Design review of the part built by this model. Coordinates are the model's own, in mm. Give positions to 0.01 mm unless a question says otherwise; leave off trailing zeros. Order: outer loops, then holes, each group sorted by start corner. A loop starts at its lowest first (then second) coordinate and runs counter-clockwise, first axis right, second up.
```python
from build123d import *

# Parameters (mm, degrees)
SKETCH1_W           = 125
SKETCH1_H           = 200
BOSS_EXTRUDE1_DEPTH = 3.175
SKETCH2_R           = 2.5
CUT_EXTRUDE1_DEPTH  = 3.175
SKETCH3_R           = 6.35
CUT_EXTRUDE2_DEPTH  = 3.175


with BuildPart() as part:
    # Sketch1 → Boss-Extrude1 (new body)
    with BuildSketch(Plane.XY):
        with Locations((-62.5, 100)):
            Rectangle(SKETCH1_W, SKETCH1_H)
    extrude(amount=BOSS_EXTRUDE1_DEPTH)

    # Sketch2 → Cut-Extrude1 (cut)
    with BuildSketch(Plane.XY.offset(3.175)):
        with Locations((-95, 190)):
            Circle(SKETCH2_R)
        with Locations((-30, 190)):
            Circle(SKETCH2_R)
    cut_extrude1 = extrude(amount=-CUT_EXTRUDE1_DEPTH, mode=Mode.SUBTRACT)

    # Mirror1: Cut-Extrude1 across plane
    add(cut_extrude1.mirror(Plane.ZX.offset(100)), mode=Mode.SUBTRACT)

    # Sketch3 → Cut-Extrude2 (cut)
    with BuildSketch(Plane.XY.offset(3.175)):
        with Locations((-62.5, 100)):
            Circle(SKETCH3_R)
    extrude(amount=-CUT_EXTRUDE2_DEPTH, mode=Mode.SUBTRACT)


solid = part.part
```
1. For pin 1 (3 mm diameter, centred on x = -95, y = 10, fed in from -Z); pin 2 (20.5 mm diameter, centred on x = -62.5, y = 100, fed in from -Z), all flat-tipped, find the tip position at first contact; note any pin that passes through.
Recorded:
pin 1: passes through
pin 2: stops at z = 0
2. Take a section at A-A (x = -95). State the section outline as (y, z) points (3 decimals), then the cut area to 3 significant figures.
Recorded:
outline: (0, 0) - (7.5, 0) - (7.5, 3.175) - (0, 3.175) - close; (12.5, 0) - (187.5, 0) - (187.5, 3.175) - (12.5, 3.175) - close; (192.5, 0) - (200, 0) - (200, 3.175) - (192.5, 3.175) - close
area: 603 mm2
3. For line 1 along Y through (x, z) = (-30, 1.6); line 2 along X through (y, z) = (10, 1.45); line 3 along Y through (x, z) = (-31.5, 1.35), list the stretches that pass through material, from the lowest coordinate up.
Recorded:
line 1: y = 0 to 7.5, 12.5 to 187.5, 192.5 to 200
line 2: x = -125 to -97.5, -92.5 to -32.5, -27.5 to 0
line 3: y = 0 to 8, 12 to 188, 192 to 200
4. Take a section at D-D (x = -62.5). State the section outline as (y, z) points (3 decimals), then the cut area to 3 significant figures.
Recorded:
outline: (0, 0) - (93.65, 0) - (93.65, 3.175) - (0, 3.175) - close; (106.35, 0) - (200, 0) - (200, 3.175) - (106.35, 3.175) - close
area: 595 mm2
5. Draft analysis for pull direction X (two halves, no side actions). For faces 1 (the face through (-30.33, 192.48, 1.61)), 2 (the face through (-77, 101, 3.175)), state which applies: pulls with the +X half, pulls with the -X half, needs draft (parallel to the pull), parting line crosses it, or undercut.
Recorded:
face 1: undercut
face 2: needs draft
6. Take a section at B-B (y = 100). State the section outline as (x, z) points (3 decimals).
Recorded:
outline: (-125, 0) - (-68.85, 0) - (-68.85, 3.175) - (-125, 3.175) - close; (-56.15, 0) - (0, 0) - (0, 3.175) - (-56.15, 3.175) - close
7. Take a section at C-C (y = 10). State the section outline as (x, z) points (3 decimals).
Recorded:
outline: (-125, 0) - (-97.5, 0) - (-97.5, 3.175) - (-125, 3.175) - close; (-92.5, 0) - (-32.5, 0) - (-32.5, 3.175) - (-92.5, 3.175) - close; (-27.5, 0) - (0, 0) - (0, 3.175) - (-27.5, 3.175) - close
